Design review of the part built by this model. Coordinates are the model's own, in mm. A direction names the side the tool comes from. Coordinates: 2 decimals unless noted, no trailing zeros. Write each loop counter-clockwise with the first axis right and the second up, starting at its lowest first coordinate (ties: lowest second). Pieces come first, ordered by that corner, then holes. Notation, with made-up numbers: M -32,-33 L -27,-33 A12 ccw -27,-11 Z; hole C 4.25,-24 d6. An arc over 180 degrees is marked long. Write item = value, one per line.
```python
from build123d import *

# Parameters (mm, degrees)
F0_W     = 60
F0_H     = 60
F1_DEPTH = 80
F2_R     = 22.5
F3_DEPTH = 80
F4_W     = 15
F4_H     = 40
F5_DEPTH = 60


with BuildPart() as f1:
    # F0 (on Top) → F1 (new body)
    with BuildSketch(Plane.XY):
        Rectangle(F0_W, F0_H)
    extrude(amount=F1_DEPTH)

    # F2 (on face) → F3 (cut)
    with BuildSketch(Plane.XY.offset(80)):
        Circle(F2_R)
    extrude(amount=-F3_DEPTH, mode=Mode.SUBTRACT)

    # F4 (on face) → F5 (cut)
    with BuildSketch(Plane.YZ.offset(30)):
        with Locations((0, 60)):
            Rectangle(F4_W, F4_H)
    extrude(amount=-F5_DEPTH, mode=Mode.SUBTRACT)


solid = f1.part
```
Q1. Consider section D-D, the plane z = 21. State the section outline as (x, y) points.
Check result:
outline = M -30,-30 L 30,-30 L 30,30 L -30,30 Z; hole C 0,0 d45
Q2. Consider section A-A, the plane y = 0. State the section outline as (x, z) points.
Check result:
outline = M -30,0 L -22.5,0 L -22.5,40 L -30,40 Z; M 22.5,0 L 30,0 L 30,40 L 22.5,40 Z
Q3. Consider section C-C, the plane x = 0. State the section outline as (y, z) points, and give its area (3 significant figures).
Check result:
outline = M -30,0 L -22.5,0 L -22.5,80 L -30,80 Z; M 22.5,0 L 30,0 L 30,80 L 22.5,80 Z
area = 1,200 mm²
Q4. Wall thickness on line 1 (Y direction, x = 0.5, z = 50.5); line 2 (X direction, y = 0, z = 23); line 3 (Y direction, x = 23, z = 63): over which ranges is each line inside the solid? List them lowest first.
Check result:
line_1 = -30 to -22.49, 22.49 to 30
line_2 = -30 to -22.5, 22.5 to 30
line_3 = -30 to -7.5, 7.5 to 30
Q5. Machinability: for faces 1 (the flat face through (-14, 20, 0)), 2 (the flat face through (26, -7.5, 60)), which of the approach directions +Z, -Z, +X, -X, +Y, -Y give a long, thin tool a straight path to every point of the face, cutting with its end or side? Answer none if there is none.
Check result:
face_1 = -Z, +X, -X, +Y, -Y
face_2 = +Z, +X, -X
Q6. For P1, Ø7, axis at x = -24, y = -2.5, coming from the +Z side; P2, Ø8, axis at x = 1.5, y = -23.5, coming from the -Z side, all flat-tipped, find the tip position at first contact; note any pin that passes through.
Check result:
P1 = 40
P2 = 0
Q7. Consider section B-B, the plane z = 72. State the section outline as (x, y) points, and give its area (3 significant figures).
Check result:
outline = M -30,-30 L 30,-30 L 30,-7.5 L 21.21,-7.5 A22.5 cw -21.21,-7.5 L -30,-7.5 Z; M -30,7.5 L -21.21,7.5 A22.5 cw 21.21,7.5 L 30,7.5 L 30,30 L -30,30 Z
area = 1,770 mm²
Q8. The part is to be moulded in two halves that separate along Y. For faces 3 (the flat face through (0, -30, 39)), 4 (the flat face through (-26, -7.5, 60)), 5 (the flat face through (-26, 0, 40)), 6 (the flat face through (30, 0, 39)), say which applies: +Y half, -Y half, draft (parallel to the pull), parting line (faces both ways), or undercut.
Check result:
face_3 = -Y half
face_4 = undercut
face_5 = undercut
face_6 = draft
